```python
from build123d import *

# Parameters (mm, degrees)
BOSS_EXTRUDE1_DEPTH  = 35.5
SKETCH2_R            = 2.15
CUT_EXTRUDE1_DEPTH   = 35.5
SKETCH3_R            = 11.25
CUT_EXTRUDE2_DEPTH   = 35.5
M3_CLEARANCE_HOLE1_D = 3.4
SKETCH8_W            = 19
SKETCH8_H            = 35.5
CUT_EXTRUDE3_DEPTH   = 16.5
CHAMFER1_SIZE        = 1.1
CHAMFER1_SIZE_2      = 12.573057533
SKETCH9_W            = 9.25
SKETCH9_H            = 16.5
CUT_EXTRUDE4_DEPTH   = 10
CHAMFER4_SIZE        = 2
CHAMFER6_SIZE        = 1
CHAMFER7_SIZE        = 0.4
CHAMFER8_SIZE        = 2


with BuildPart() as part:
    # Sketch1 → Boss-Extrude1 (new body)
    with BuildSketch(Plane.XY):
        Polygon((0, 0), (0, -10), (9.25, -10), (9.25, -26.5), (44.75, -26.5), (44.75, -10), (54, -10), (54, 0), align=None)
    extrude(amount=BOSS_EXTRUDE1_DEPTH)

    # Sketch2 → Cut-Extrude1 (cut)
    with BuildSketch(Plane.XY.offset(35.5)):
        with Locations((4.5, -5)):
            Circle(SKETCH2_R)
        with Locations((49.5, -5)):
            Circle(SKETCH2_R)
    extrude(amount=-CUT_EXTRUDE1_DEPTH, mode=Mode.SUBTRACT)

    # Sketch3 → Cut-Extrude2 (cut)
    with BuildSketch(Plane.XZ.offset(26.5)):
        with Locations((27, 17.75)):
            Circle(SKETCH3_R)
    extrude(amount=-CUT_EXTRUDE2_DEPTH, mode=Mode.SUBTRACT)

    # M3 Clearance Hole1 (through all)
    with Locations(Plane(origin=(0, -26.5, 0), x_dir=(-1, 0, 0), z_dir=(0, -1, 0))):
        with Locations((-14, -30.75), (-40, -30.75), (-40, -4.75), (-14, -4.75)):
            Hole(M3_CLEARANCE_HOLE1_D / 2)

    # Sketch8 → Cut-Extrude3 (cut)
    with BuildSketch(Plane.XZ.offset(26.5)):
        with Locations((27, 17.75)):
            Rectangle(SKETCH8_W, SKETCH8_H)
    extrude(amount=-CUT_EXTRUDE3_DEPTH, mode=Mode.SUBTRACT)

    # Chamfer1
    # the kernel refuses this chamfer: 12.573057533, 1.1 mm, written as the material it takes off along each edge
    with BuildSketch(Plane(origin=(36.5, -59.185348851, 0), x_dir=(0.9159861691531063, 0, -0.40120984275091887), z_dir=(0, 1, 0)), Plane(origin=(17.5, -59.185348851, 35.5), x_dir=(-0.9159861691531072, 0, 0.40120984275091703), z_dir=(0, 1, 0))) as chamfer1_piece_1:
        Polygon((CHAMFER1_SIZE * 0.915986169153, -CHAMFER1_SIZE * 0.401209842751), (-CHAMFER1_SIZE_2 * 0.401209842752, -CHAMFER1_SIZE_2 * 0.915986169156), (0, 0), align=None)
    extrude(amount=49.185348851, mode=Mode.SUBTRACT)
    with BuildSketch(Plane(origin=(17.5, -59.185348851, 0), x_dir=(-0.9159861691531066, 0, -0.4012098427509178), z_dir=(0, 1, 0)), Plane(origin=(36.5, -59.185348851, 35.5), x_dir=(0.9159861691531066, 0, 0.40120984275091803), z_dir=(0, 1, 0))) as chamfer1_piece_2:
        Polygon((CHAMFER1_SIZE * 0.915986169153, CHAMFER1_SIZE * 0.401209842751), (-CHAMFER1_SIZE_2 * 0.401209842752, CHAMFER1_SIZE_2 * 0.915986169156), (0, 0), align=None)
    extrude(amount=49.185348851, mode=Mode.SUBTRACT)

    # Sketch9 → Cut-Extrude4 (cut)
    with BuildSketch(Plane(origin=(0, 0, 0), x_dir=(1, 0, 0), z_dir=(0, 1, 0))):
        with Locations((4.625, -17.75)):
            Rectangle(SKETCH9_W, SKETCH9_H)
        with Locations((49.375, -17.75)):
            Rectangle(SKETCH9_W, SKETCH9_H)
    extrude(amount=-CUT_EXTRUDE4_DEPTH, mode=Mode.SUBTRACT)

    # Chamfer4
    chamfer4_edges = [part.edges().sort_by_distance(p)[0] for p in [
        (54, 0, 30.75),
        (54, -10, 30.75),
        (0, -10, 30.75),
        (0, 0, 30.75),
        (54, 0, 4.75),
        (54, -10, 4.75),
        (0, -10, 4.75),
        (0, 0, 4.75),
    ]]
    chamfer(chamfer4_edges, length=CHAMFER4_SIZE)

    # Chamfer6
    chamfer6_edges = [part.edges().sort_by_distance(p)[0] for p in [
        (15.75, 0, 17.75),
        (37.820600651, -26.5, 14.67150986),
        (15.75, -26.5, 17.75),
    ]]
    chamfer(chamfer6_edges, length=CHAMFER6_SIZE)

    # Chamfer7
    chamfer7_edges = [part.edges().sort_by_distance(p)[0] for p in [
        (2.35, -5, 9.5),
        (2.35, -5, 26),
        (47.35, -5, 26),
        (47.35, -5, 9.5),
        (2.35, -5, 0),
        (2.35, -5, 35.5),
        (47.35, -5, 0),
        (47.35, -5, 35.5),
        (12.3, -26.5, 4.75),
        (12.3, 0, 4.75),
        (38.3, -26.5, 4.75),
        (38.3, 0, 4.75),
        (38.3, -26.5, 30.75),
        (38.3, 0, 30.75),
        (12.3, -26.5, 30.75),
        (12.3, 0, 30.75),
    ]]
    chamfer(chamfer7_edges, length=CHAMFER7_SIZE)

    # Chamfer8
    chamfer8_edges = [part.edges().sort_by_distance(p)[0] for p in [
        (9.25, -18.25, 35.5),
        (44.75, -18.25, 35.5),
        (44.75, -18.25, 0),
        (9.25, -18.25, 0),
    ]]
    chamfer(chamfer8_edges, length=CHAMFER8_SIZE)


solid = part.part
```
Work out the finished part from the listing and answer in its coordinate system (mm). A direction names the side the tool comes from. Round coordinates to 2 decimals unless told otherwise and drop trailing zeros. Loops run counter-clockwise (first coordinate to the right, second up) from the corner with the lowest first, then second, coordinate; pieces in that order, holes last.
(1) For faces 4 (the cylindrical face through (38.65, -13.07, 31.78)), 5 (the flat face through (43.76, -18.37, 34.49)), determine the directions among +Z, -Z, +X, -X, +Y, -Y from which every point of the face is accessible in a straight line to the end or side of a thin tool.
Computed values:
face 4: +Y, -Y
face 5: +Z, +X, -Y
(2) The part is cut by section C-C, the plane z = 30.75. Give the number of separate pieces and of enclosed holes in the cut face, and give its area (3 significant figures).
Computed values:
separate pieces: 3
enclosed holes: 2
area: 572 mm2
(3) This flat-tipped pin is pushed along its axis until it touches: P1, Ø4.5, axis at x = 4.5, z = 30.5, coming from the -Y side. Where does it stop, or does it pass through?
Computed values:
P1: stops at y = -10
(4) The part is cut by section D-D, the plane x = 49.5. Give the vertices of the cut face in (y, z).
Computed values:
outline: (-10, 0) - (-7.55, 0) - (-7.15, 0.4) - (-7.15, 9.1) - (-7.55, 9.5) - (-10, 9.5) - close; (-10, 26) - (-7.55, 26) - (-7.15, 26.4) - (-7.15, 35.1) - (-7.55, 35.5) - (-10, 35.5) - close; (-2.85, 0.4) - (-2.45, 0) - (0, 0) - (0, 9.5) - (-2.45, 9.5) - (-2.85, 9.1) - close; (-2.85, 26.4) - (-2.45, 26) - (0, 26) - (0, 35.5) - (-2.45, 35.5) - (-2.85, 35.1) - close
(5) The part is cut by section A-A, the plane y = -21.75. Give the vertices of the cut face in (x, z).
Computed values:
outline: (9.25, 2) - (11.25, 0) - (16.4, 0) - (17.43, 11.83) arc R11.25 cw to (17.43, 23.67) - (16.4, 35.5) - (11.25, 35.5) - (9.25, 33.5) - close; (36.57, 11.83) - (37.6, 0) - (42.75, 0) - (44.75, 2) - (44.75, 33.5) - (42.75, 35.5) - (37.6, 35.5) - (36.57, 23.67) arc R11.25 cw to start; hole circle Ø3.4 at (14, 4.75); hole circle Ø3.4 at (14, 30.75); hole circle Ø3.4 at (40, 4.75); hole circle Ø3.4 at (40, 30.75)
(6) The mould has two halves that part along Z. Classify faces 1 (the cylindrical face through (38.65, -13.07, 5.78)), 2 (the flat face through (54, -5, 5)), 3 (the flat face through (16.91, -18.37, 5.83)): pulls with the +Z half, pulls with the -Z half, needs draft (parallel to the pull), parting line crosses it, or undercut.
Computed values:
face 1: undercut
face 2: needs draft
face 3: pulls with the -Z half
(7) Find the intervals of material crossed by L1, parallel to Z at x = 14, y = -19.25; L2, parallel to X at y = -3.5, z = 18; L3, parallel to Z at x = 52, y = -7.5, in increasing order.
Computed values:
L1: z = 0 to 3.05, 6.45 to 29.05, 32.45 to 35.5
L2: x = 9.25 to 15.75, 38.25 to 44.75
L3: z = 0 to 9.5, 26 to 35.5
(8) The part is cut by section B-B, the plane x = 27. Give the vertices of the cut face in (y, z), and give its area (3 significant figures).
Computed values:
outline: (-10, 0) - (0, 0) - (0, 5.5) - (-1, 6.5) - (-10, 6.5) - close; (-10, 29) - (-1, 29) - (0, 30) - (0, 35.5) - (-10, 35.5) - close
area: 129 mm2
